```python
from build123d import *

# Parameters (mm, degrees)
F1_DEPTH = 5
F2_W     = 40
F2_H     = 40
F3_DEPTH = 10
F5_DEPTH = 10
F7_DEPTH = 10


with BuildPart() as f1:
    # F0 (on Front) → F1 (new body, symmetric)
    with BuildSketch(Plane.XZ):
        with BuildLine():
            ThreePointArc((-20, -15), (0, -35), (20, -15))
            Line((20, -15), (9, -15))
            ThreePointArc((9, -15), (0, -24), (-9, -15))
            Line((-9, -15), (-20, -15))
        make_face()
        with BuildLine():
            Line((9, -15), (20, -15))
            Line((20, -15), (20, 15))
            Line((20, 15), (-20, 15))
            Line((-20, 15), (-20, -15))
            Line((-20, -15), (-9, -15))
            ThreePointArc((-9, -15), (0, -6), (9, -15))
        make_face()
    extrude(amount=F1_DEPTH, both=True)

    # F2 (on face) → F3 (join)
    with BuildSketch(Plane.XY.offset(15)):
        Rectangle(F2_W, F2_H)
    extrude(amount=F3_DEPTH)

    # F4 (on face) → F5 (join)
    with BuildSketch(Plane.XZ.offset(20)):
        with BuildLine():
            ThreePointArc((-9, 45), (0, 54), (9, 45))
            Line((9, 45), (20, 45))
            ThreePointArc((20, 45), (0, 65), (-20, 45))
            Line((-20, 45), (-9, 45))
        make_face()
        with BuildLine():
            Line((20, 45), (9, 45))
            ThreePointArc((9, 45), (0, 36), (-9, 45))
            Line((-9, 45), (-20, 45))
            Line((-20, 45), (-20, 25))
            Line((-20, 25), (20, 25))
            Line((20, 25), (20, 45))
        make_face()
    extrude(amount=-F5_DEPTH)

    # F6 (on face) → F7 (join)
    with BuildSketch(Plane(origin=(0, 20, 0), x_dir=(-1, 0, 0), z_dir=(0, 1, 0))):
        with BuildLine():
            ThreePointArc((-9, 45), (0, 54), (9, 45))
            Line((9, 45), (20, 45))
            ThreePointArc((20, 45), (0, 65), (-20, 45))
            Line((-20, 45), (-9, 45))
        make_face()
        with BuildLine():
            Line((20, 45), (9, 45))
            ThreePointArc((9, 45), (0, 36), (-9, 45))
            Line((-9, 45), (-20, 45))
            Line((-20, 45), (-20, 25))
            Line((-20, 25), (20, 25))
            Line((20, 25), (20, 45))
        make_face()
    extrude(amount=-F7_DEPTH)


solid = f1.part
```
Verification items for the finished model (mm, model axes). A direction names the side the tool comes from. Coordinates: 2 decimals unless noted, no trailing zeros. Loops run counter-clockwise (first coordinate to the right, second up) from the corner with the lowest first, then second, coordinate; pieces in that order, holes last. Notation, with made-up numbers: (86, -23.5) -> (110, -23.5) arc R24 cw to (110, 12.5) -> close; hole circle Ø11 at (10, 59). An arc over 180 degrees is marked (long way). Put each result on its own line as item: value.
1. Section check C-C, the plane y = -11. Record the boundary of the cut face in (x, z), then the cut area to 3 significant figures.
Result set:
outline: (-20, 15) -> (20, 15) -> (20, 45) arc R20 ccw to (-20, 45) -> close; hole circle Ø18 at (0, 45)
area: 1,570 mm^2
2. Section check A-A, the plane x = 0. Record the boundary of the cut face in (y, z).
Result set:
outline: (-20, 15) -> (-5, 15) -> (-5, -6) -> (5, -6) -> (5, 15) -> (20, 15) -> (20, 36) -> (10, 36) -> (10, 25) -> (-10, 25) -> (-10, 36) -> (-20, 36) -> close; (-20, 54) -> (-10, 54) -> (-10, 65) -> (-20, 65) -> close; (-5, -35) -> (5, -35) -> (5, -24) -> (-5, -24) -> close; (10, 54) -> (20, 54) -> (20, 65) -> (10, 65) -> close
3. Tool access check on faces 4 (the face through (0, 13, 15)), 5 (the face through (1.172, 15.07, 36.077)), 6 (the face through (0, -5, -4)), 7 (the face through (0, 0, -35)), 8 (the face through (-4, 10, 36)). Record the directions out of +Z, -Z, +X, -X, +Y, -Y that give a thin tool (end or side, any length) a straight path to the whole face; none if there is none.
Result set:
face 4: -Z, +X, -X, +Y
face 5: +Y, -Y
face 6: -Z, +X, -X, -Y
face 7: -Z, +Y, -Y
face 8: +Z, +X, -X
4. Thickness scan on line 1 (Z direction, x = 0, y = 15); line 2 (Z direction, x = 0, y = -2.25); line 3 (X direction, y = -14, z = 45). Record the ranges inside material, lowest first.
Result set:
line 1: z = 15 to 36, 54 to 65
line 2: z = -35 to -24, -6 to 25
line 3: x = -20 to -9, 9 to 20
5. Gauge pin test, flat ends, axial feed: P1, Ø4, axis at x = -3.5, y = -3.5, coming from the +Z side; P2, Ø12, axis at x = 2.5, y = 10.5, coming from the -Z side; P3, Ø5, axis at x = -1, z = -4, coming from the -Y side. Record the tip position at first contact, or that the pin passes through.
Result set:
P1: stops at z = 25
P2: stops at z = -35
P3: stops at y = -5
6. Section check D-D, the plane x = 16. Record the boundary of the cut face in (y, z).
Result set:
outline: (-20, 15) -> (-5, 15) -> (-5, -27) -> (5, -27) -> (5, 15) -> (20, 15) -> (20, 57) -> (10, 57) -> (10, 25) -> (-10, 25) -> (-10, 57) -> (-20, 57) -> close
7. Section check B-B, the plane z = 38. Record the boundary of the cut face in (x, y).
Result set:
outline: (-20, -20) -> (-5.66, -20) -> (-5.66, -10) -> (-20, -10) -> close; (-20, 10) -> (-5.66, 10) -> (-5.66, 20) -> (-20, 20) -> close; (5.66, -20) -> (20, -20) -> (20, -10) -> (5.66, -10) -> close; (5.66, 10) -> (20, 10) -> (20, 20) -> (5.66, 20) -> close
8. Mould release check, pull along Z, two halves, no side actions. Record for faces 1 (the face through (0, 15, 65)), 2 (the face through (-4.153, -0.07, -22.985)), 3 (the face through (0, -20, 35)): pulls with the +Z half, pulls with the -Z half, needs draft (parallel to the pull), parting line crosses it, or undercut.
Result set:
face 1: pulls with the +Z half
face 2: undercut
face 3: needs draft
